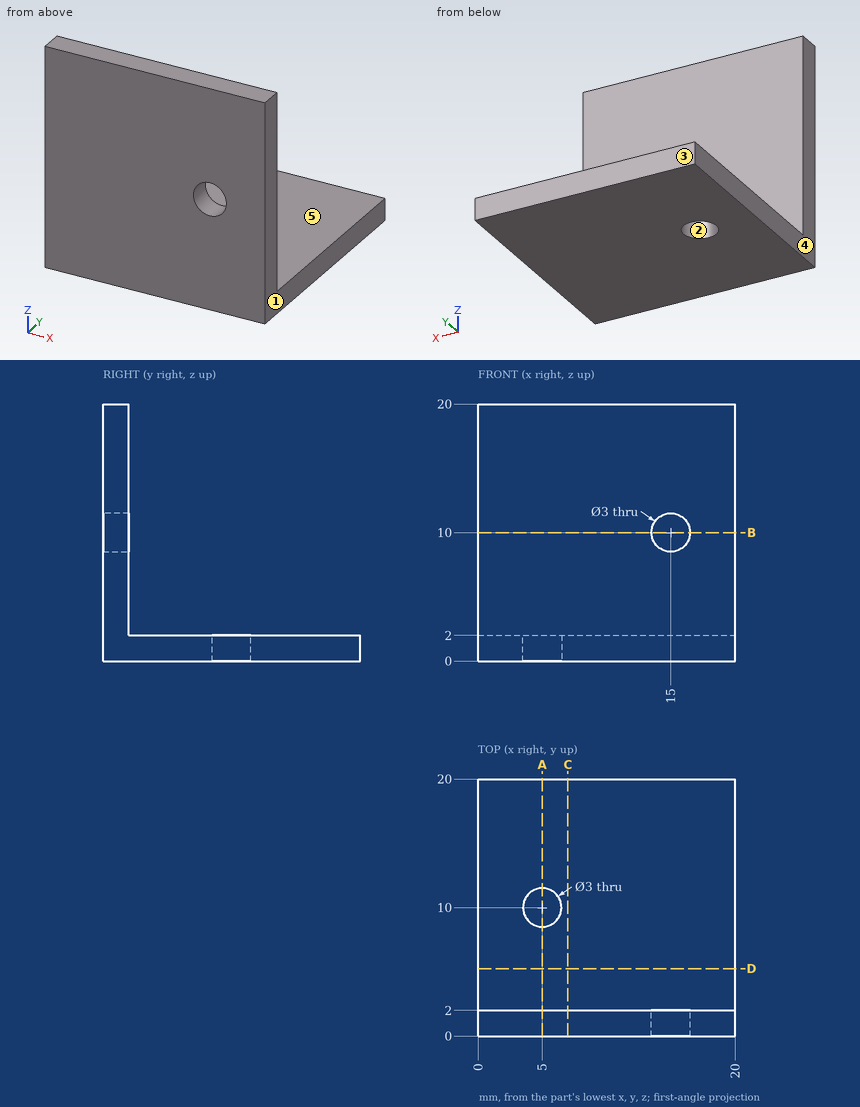
Could you check a few things on this drawing? It's one solid part, dimensions in mm from its lowest x, y, z. A direction names the side the tool comes from. Coordinates: 2 decimals unless noted, no trailing zeros. Write each loop counter-clockwise with the first axis right and the second up, starting at its lowest first coordinate (ties: lowest second). Pieces come first, ordered by that corner, then holes. Notation, with made-up numbers: (54, -38.5) - (94, -38.5) arc R24 ccw to (94, -24.5) - close; hole circle Ø5 at (64.5, -32). An arc over 180 degrees is marked (long way). Put each result on its own line as item: value. Start each with the question number.
Q1. I want a section at A-A on x = 5. Write out the boundary of the cut face in (y, z), plus the area to 3 significant figures.
Q2. Which directions (+Z, -Z, +X, -X, +Y, -Y) give clear straight access to the entire face, cutting with the end or side of a thin tool? Please do the marked faces 4 and 5.
Q3. Thinking about a two-plate mould opening in X: for the marked faces 1, 2 and 3, which applies, pulls with the +X half, pulls with the -X half, needs draft (parallel to the pull), parting line crosses it, or undercut?
Q4. I'm going to push a flat-ended pin straight in: P1, Ø5, axis at x = 4, y = 14, coming from the +Z side. Where does the tip first touch, or does it pass through?
Q5. I want a section at D-D on y = 5.25. Write out the boundary of the cut face in (x, z), plus the area to 3 significant figures.
Q6. I want a section at B-B on z = 10. Write out the boundary of the cut face in (x, y), plus the area to 3 significant figures.
Q7. Please list where these lines run through material, in increasing order: L1, parallel to X at y = 1.35, z = 10; L2, parallel to Z at x = 7.25, y = 5.5.
Q8. I want a section at C-C on x = 7. Write out the boundary of the cut face in (y, z).
Checks:
1. outline: (0, 0) - (8.5, 0) - (8.5, 2) - (2, 2) - (2, 20) - (0, 20) - close; (11.5, 0) - (20, 0) - (20, 2) - (11.5, 2) - close
1. area: 70.0 mm²
2. face 4: +Z, -Z, -X, +Y, -Y
2. face 5: +Z, +X, -X, +Y
3. face 1: pulls with the +X half
3. face 2: undercut
3. face 3: needs draft
4. P1: z = 2
5. outline: (0, 0) - (20, 0) - (20, 2) - (0, 2) - close
5. area: 40.0 mm²
6. outline: (0, 0) - (13.5, 0) - (13.5, 2) - (0, 2) - close; (16.5, 0) - (20, 0) - (20, 2) - (16.5, 2) - close
6. area: 34.0 mm²
7. L1: 0 to 13.5, 16.5 to 20
7. L2: 0 to 2
8. outline: (0, 0) - (20, 0) - (20, 2) - (2, 2) - (2, 20) - (0, 20) - close
